Verification items for this drawing (mm, ordinates from the low corner). Coordinates: 2 decimals unless noted, no trailing zeros. Order: outer loops, then holes, each group sorted by start corner. A loop starts at its lowest first (then second) coordinate and runs counter-clockwise, first axis right, second up. Notation, with made-up numbers: (76.25, 44) -> (126.25, 44) arc R33 cw to (126.25, 78) -> close; hole circle Ø3 at (24.5, 86). An arc over 180 degrees is marked (long way). Write each question's results on one line, items separated by ' | '. Start each with the question number.
(1) Draft check along Y on the marked faces 1, 2 and 3. Enter one of: +Y half, -Y half, draft (parallel to the pull), parting line (faces both ways), or undercut.
(2) Go/stop test with flat-tipped pins: pin 1 (3 mm diameter, centred on x = 8.5, y = 5, fed in from +Z); pin 2 (2 mm diameter, centred on y = 10.5, z = 5.5, fed in from -X); pin 3 (2 mm diameter, centred on y = 6, z = 3, fed in from +X); pin 4 (3 mm diameter, centred on x = 4.5, z = 2, fed in from -Y). Record where each tip stops, or that it passes through.
(3) Cross-section at A-A on y = 12. Enter the section's corners in (x, z).
(4) Cross-section at C-C on z = 4. Enter the section's corners in (x, y), and give its area (3 significant figures).
(5) Thickness scan on probe 1 along Y at (x, z) = (12, 5); probe 2 along X at (y, z) = (18.25, 6.75). Record the ranges inside material, lowest first. Write a range as [from, to].
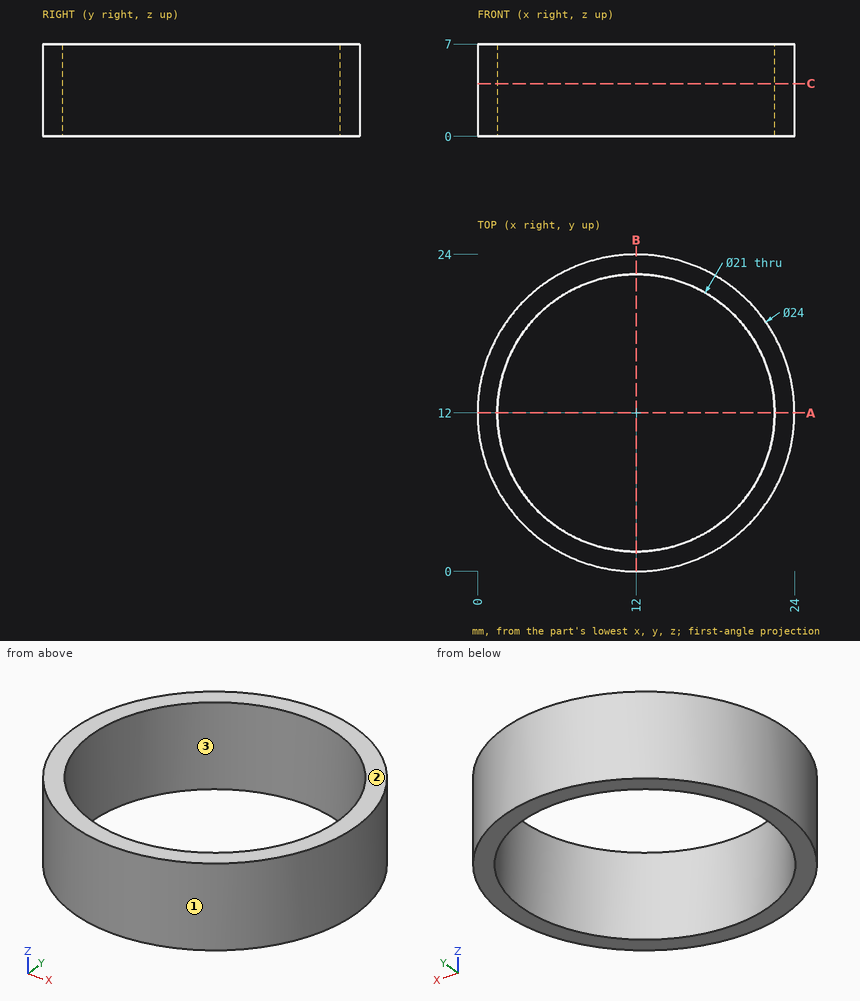
Results are:
1) face 1: parting line | face 2: draft | face 3: undercut
2) pin 1: passes through | pin 2: stops at x = 0.01 | pin 3: stops at x = 22.91 | pin 4: stops at y = 1.61
3) outline: (0, 0) -> (1.5, 0) -> (1.5, 7) -> (0, 7) -> close; (22.5, 0) -> (24, 0) -> (24, 7) -> (22.5, 7) -> close
4) outline: circle Ø24 at (12, 12); hole circle Ø21 at (12, 12) | area: 106 mm2
5) probe 1: y = [0, 1.5], [22.5, 24] | probe 2: x = [1.76, 3.56], [20.44, 22.24]
